Geometry check sheet. Reference: the model listing, model coordinates, mm. Face numbers are marked on the shaded views. A direction names the side the tool comes from. Round coordinates to 2 decimals unless told otherwise and drop trailing zeros. Order: outer loops, then holes, each group sorted by start corner. A loop starts at its lowest first (then second) coordinate and runs counter-clockwise, first axis right, second up.
(1) Cross-section at A-A on z = 3.75. Enter the section's corners in (x, y), and give its area (3 significant figures).
(2) Thickness scan on L1, parallel to Y at x = 35, z = 8.5; L2, parallel to Y at x = 3.5, z = 2.25; L3, parallel to X at y = -6.5, z = 9. Record the ranges inside material, lowest first.
(3) Cross-section at D-D on y = -3.5. Enter the section's corners in (x, z).
(4) Cross-section at B-B on x = 29.5. Enter the section's corners in (y, z), and give its area (3 significant figures).
(5) Cross-section at C-C on z = 9. Enter the section's corners in (x, y).
(6) Set-up check for the marked faces 1 and 2: record each of +Z, -Z, +X, -X, +Y, -Y from which the full face is reachable in a straight line by a thin tool's end or side.
(7) Gauge pin test, flat ends, axial feed: P1, Ø0.8, axis at y = 1, z = 3.5, coming from the +X side; P2, Ø3, axis at x = 14.5, z = 7.5, coming from the +Y side; P3, Ø4, axis at y = -14, z = 10, coming from the +X side. Record the tip position at first contact, or that the pin passes through.
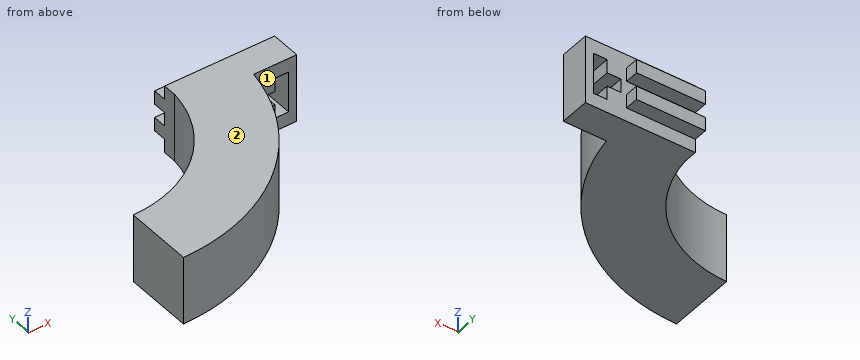
from build123d import *

# Parameters (mm, degrees)
SKETCH1_R               = 35
SKETCH1_R_2             = 22.3
BOSS_EXTRUDE2_DEPTH     = 12.7
SKETCH4_W               = 2.54
SKETCH4_H               = 76.791301982
SKETCH4_W_2             = 87.412375573
SKETCH4_H_2             = 2.54
CUT_EXTRUDE_THIN4_DEPTH = 12.7
SKETCH7_W               = 12.775704106
SKETCH7_H               = 12.7
BOSS_EXTRUDE3_DEPTH     = 2.54
SKETCH11_W              = 12.775704106
SKETCH11_H              = 2.54
SKETCH11_W_2            = 12.761411891
BOSS_EXTRUDE6_DEPTH     = 2.54
SKETCH12_W              = 12.7
SKETCH12_H              = 5.594236833
BOSS_EXTRUDE7_DEPTH     = 7.62
SKETCH12_2_W            = 12.7
SKETCH12_2_H            = 5.594236833
BOSS_EXTRUDE8_DEPTH     = 2.54
CAVITY3_START           = 38.513729061
CAVITY3_OUTLINE_W       = 5.594236833
CAVITY3_OUTLINE_H       = 7.62
CAVITY3_DEPTH           = 2.54
CAVITY3_START_2         = 35.973729061
CAVITY3_2_OUTLINE_W     = 5.594236833
CAVITY3_2_OUTLINE_H     = 2.54
CAVITY3_2_DEPTH         = 2.54


# Read off the part's stored shape, not the designer's step: Cavity3
with BuildPart() as part:
    # Sketch1 → Boss-Extrude2 (new body)
    with BuildSketch(Plane.XY):
        Circle(SKETCH1_R)
        Circle(SKETCH1_R_2, mode=Mode.SUBTRACT)
    extrude(amount=BOSS_EXTRUDE2_DEPTH)

    # Sketch4 → Cut-Extrude-Thin4 (cut)
    with BuildSketch(Plane.XY.offset(12.7)):
        with Locations((-1.27, -1.456872926)):
            Rectangle(SKETCH4_W, SKETCH4_H)
        with Locations((4.088643373, -1.27)):
            Rectangle(SKETCH4_W_2, SKETCH4_H_2)
    extrude(amount=-CUT_EXTRUDE_THIN4_DEPTH, mode=Mode.SUBTRACT)


with BuildPart() as body_2:
    # of the pieces the cut leaves, the one that is kept (cut_extrude_thin4_keep)
    add(part.part.solids().sort_by_distance((34.907712615, -2.54, 12.7))[0])

    # Sketch7 → Boss-Extrude3 (add)
    with BuildSketch(Plane(origin=(0, -2.54, 0), x_dir=(1, 0, 0), z_dir=(0, 1, 0))):
        with Locations((28.542725106, -6.35)):
            Rectangle(SKETCH7_W, SKETCH7_H)
    extrude(amount=BOSS_EXTRUDE3_DEPTH)

    # Sketch11 → Boss-Extrude6 (add)
    with BuildSketch(Plane(origin=(0, 0, 0), x_dir=(1, 0, 0), z_dir=(0, 1, 0))):
        with Locations((28.542725106, -3.81)):
            Rectangle(SKETCH11_W, SKETCH11_H)
        with Locations((28.535578999, -8.89)):
            Rectangle(SKETCH11_W_2, SKETCH11_H)
    extrude(amount=BOSS_EXTRUDE6_DEPTH)

    # Sketch12 → Boss-Extrude7 (add)
    with BuildSketch(Plane(origin=(34.930577159, 0, 0), x_dir=(0, 0, -1), z_dir=(1, 0, 0))):
        with Locations((-6.35, -2.797118417)):
            Rectangle(SKETCH12_W, SKETCH12_H)
    extrude(amount=BOSS_EXTRUDE7_DEPTH)

    # Sketch12<2> → Boss-Extrude8 (add)
    with BuildSketch(Plane(origin=(34.930577159, 0, 0), x_dir=(0, 0, -1), z_dir=(1, 0, 0))):
        with Locations((-6.35, -2.797118417)):
            Rectangle(SKETCH12_2_W, SKETCH12_2_H)
    extrude(amount=-BOSS_EXTRUDE8_DEPTH)

    # Cavity3 outline → Cavity3 (cut)
    with BuildSketch(Plane.YZ.offset(CAVITY3_START)):
        with Locations((-2.797118417, 6.296394857)):
            Rectangle(CAVITY3_OUTLINE_W, CAVITY3_OUTLINE_H)
    extrude(amount=CAVITY3_DEPTH, mode=Mode.SUBTRACT)

    # Cavity3 2 outline → Cavity3 2 (cut)
    with BuildSketch(Plane.YZ.offset(CAVITY3_START_2)):
        with Locations((-2.797118417, 6.296394857)):
            Rectangle(CAVITY3_2_OUTLINE_W, CAVITY3_2_OUTLINE_H)
    extrude(amount=CAVITY3_2_DEPTH, mode=Mode.SUBTRACT)


solid = body_2.part
Found:
1. outline: (0, -35) arc R35 ccw to (34.55, -5.59) - (38.51, -5.59) - (38.51, 0) - (34.93, 0) - (34.93, 2.54) - (22.15, 2.54) - (22.15, -2.54) arc R22.3 cw to (0, -22.3) - close; (41.05, -5.59) - (42.55, -5.59) - (42.55, 0) - (41.05, 0) - close
1. area: 633 mm2
2. L1: y = -5.59 to 0
2. L2: y = -34.82 to -22.02
2. L3: x = 21.33 to 34.39
3. outline: (22.02, 0) - (42.55, 0) - (42.55, 12.7) - (22.02, 12.7) - close; hole (35.97, 5.03) - (38.51, 5.03) - (38.51, 2.49) - (41.05, 2.49) - (41.05, 10.11) - (38.51, 10.11) - (38.51, 7.57) - (35.97, 7.57) - close
4. outline: (-18.83, 0) - (0, 0) - (0, 2.54) - (2.54, 2.54) - (2.54, 5.08) - (0, 5.08) - (0, 7.62) - (2.54, 7.62) - (2.54, 10.16) - (0, 10.16) - (0, 12.7) - (-18.83, 12.7) - close
4. area: 252 mm2
5. outline: (0, -35) arc R35 ccw to (34.55, -5.59) - (38.51, -5.59) - (38.51, 0) - (34.92, 0) - (34.92, 2.54) - (22.15, 2.54) - (22.15, -2.54) arc R22.3 cw to (0, -22.3) - close; (41.05, -5.59) - (42.55, -5.59) - (42.55, 0) - (41.05, 0) - close
6. face 1: +Z, -Z, +X, -Y
6. face 2: +Z, +X, -X, +Y, -Y
7. P1: stops at x = 34.93
7. P2: stops at y = -15.53
7. P3: stops at x = 32.88
